```python
from build123d import *

# Parameters (mm, degrees)
CUT_EXTRUDE1_DEPTH  = 2.54
SKETCH3_R           = 2.413
BOSS_EXTRUDE1_DEPTH = 9.525
CHAMFER1_SIZE       = 0.762
CHAMFER1_SIZE2      = 0.439940905


with BuildPart() as part:
    # Sketch1 → Revolve1 (revolve)
    with BuildSketch(Plane(origin=(0, 0, 0), x_dir=(1, 0, 0), z_dir=(0, 1, 0))):
        with BuildLine():
            Line((0, 0), (3.71475, 0))
            ThreePointArc((3.71475, 0), (3.894355122, -0.074394878), (3.96875, -0.254))
            Line((3.96875, -0.254), (3.96875, -4.572))
            ThreePointArc((3.96875, -4.572), (3.894355122, -4.751605122), (3.71475, -4.826))
            Line((3.71475, -4.826), (0, -4.826))
            Line((0, -4.826), (0, 0))
        make_face()
    revolve(axis=Axis((0, 0, 0), (0, 0, -1)))

    # Sketch2 → Cut-Extrude1 (cut)
    with BuildSketch(Plane(origin=(0, 0, 0), x_dir=(-1, 0, 0), z_dir=(0, 0, -1))):
        Polygon((0, 2.291358881), (-1.984375, 1.14567944), (-1.984375, -1.14567944), (0, -2.291358881), (1.984375, -1.14567944), (1.984375, 1.14567944), align=None)
    extrude(amount=-CUT_EXTRUDE1_DEPTH, mode=Mode.SUBTRACT)

    # Sketch3 → Boss-Extrude1 (add)
    with BuildSketch(Plane.XY.offset(4.826)):
        with Locations(Location((0, 0, 0), (0, 0, 180))):
            Circle(SKETCH3_R)
    extrude(amount=BOSS_EXTRUDE1_DEPTH)

    # Chamfer1
    chamfer1_edges = [part.edges().sort_by_distance(p)[0] for p in [
        (2.413, 0, 14.351),
    ]]
    chamfer1_side = [part.faces().sort_by_distance(p)[0] for p in [
        (2.413, 0, 9.5885),
    ]]
    chamfer(chamfer1_edges, length=CHAMFER1_SIZE, length2=CHAMFER1_SIZE2, reference=chamfer1_side[0])


solid = part.part
```
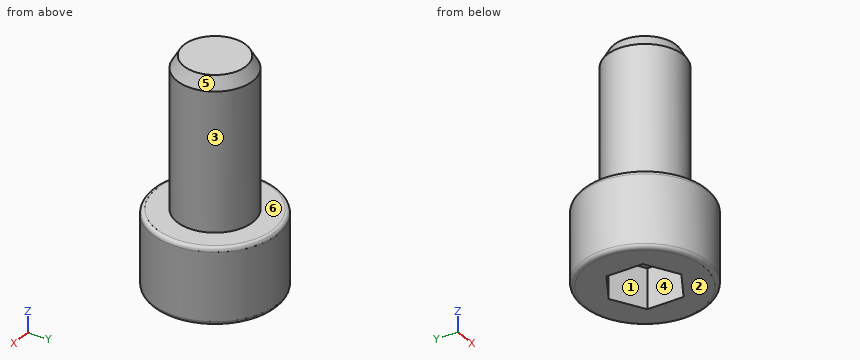
Design review of the part built by this model. Coordinates are the model's own, in mm. Face numbers are marked on the shaded views. A direction names the side the tool comes from. Coordinates: 2 decimals unless noted, no trailing zeros. Order: outer loops, then holes, each group sorted by start corner. A loop starts at its lowest first (then second) coordinate and runs counter-clockwise, first axis right, second up.
1) For the marked faces 1, 2 and 3, list the 3-axis set-ups (+Z, -Z, +X, -X, +Y, -Y) from which the entire face can be reached by the end or side of a thin tool; tool diameter is ignored.
2) Take a section at A-A, the plane y = 0. Give the boundary of the cut face in (x, z).
3) Clearance check with a flat-ended pin moving along its axis: pin 1 (2 mm diameter, centred on x = 1, z = 11, fed in from +Y). State where the tip first meets the part, or that it passes through.
4) Mouldability with a two-part tool opening along X and no side actions: class the marked faces 4, 5 and 6 as +X half, -X half, draft (parallel to the pull), parting line (faces both ways), or undercut.
5) Take a section at B-B, the plane z = 3. Give the boundary of the cut face in (x, y).
6) Wall thickness on line 1 along Z through (x, y) = (1, -2.25); line 2 along Y through (x, z) = (0, 6.25); line 3 along Y through (x, z) = (-0.5, 2.25): over which ranges is each line inside the solid? List them lowest first.
7) Take a section at C-C, the plane z = 6.75. Give the boundary of the cut face in (x, y).
Returned:
1. face 1: -Z
1. face 2: -Z, +X, -X, +Y, -Y
1. face 3: +Z
2. outline: (-3.97, 0.25) arc R0.25 ccw to (-3.71, 0) - (-1.98, 0) - (-1.98, 2.54) - (1.98, 2.54) - (1.98, 0) - (3.71, 0) arc R0.25 ccw to (3.97, 0.25) - (3.97, 4.57) arc R0.25 ccw to (3.71, 4.83) - (2.41, 4.83) - (2.41, 13.59) - (1.97, 14.35) - (-1.97, 14.35) - (-2.41, 13.59) - (-2.41, 4.83) - (-3.71, 4.83) arc R0.25 ccw to (-3.97, 4.57) - close
3. pin 1: stops at y = 2.41
4. face 4: undercut
4. face 5: parting line
4. face 6: draft
5. outline: circle Ø7.94 at (0, 0)
6. line 1: z = 0 to 4.83
6. line 2: y = -2.41 to 2.41
6. line 3: y = -3.94 to -2, 2 to 3.94
7. outline: circle Ø4.83 at (0, 0)
